Job drawing, mm, ordinate dimensions from the low corner. One solid piece. A direction names the side the tool comes from. Give positions to 0.01 mm unless a question says otherwise; leave off trailing zeros. Loops run counter-clockwise (first coordinate to the right, second up) from the corner with the lowest first, then second, coordinate; pieces in that order, holes last. Notation, with made-up numbers: M 64,7.5 L 110,7.5 A25 ccw 110,33.5 Z; hole C -34.75,88 d10. An arc over 180 degrees is marked long. Answer as CSV lines item,"result".
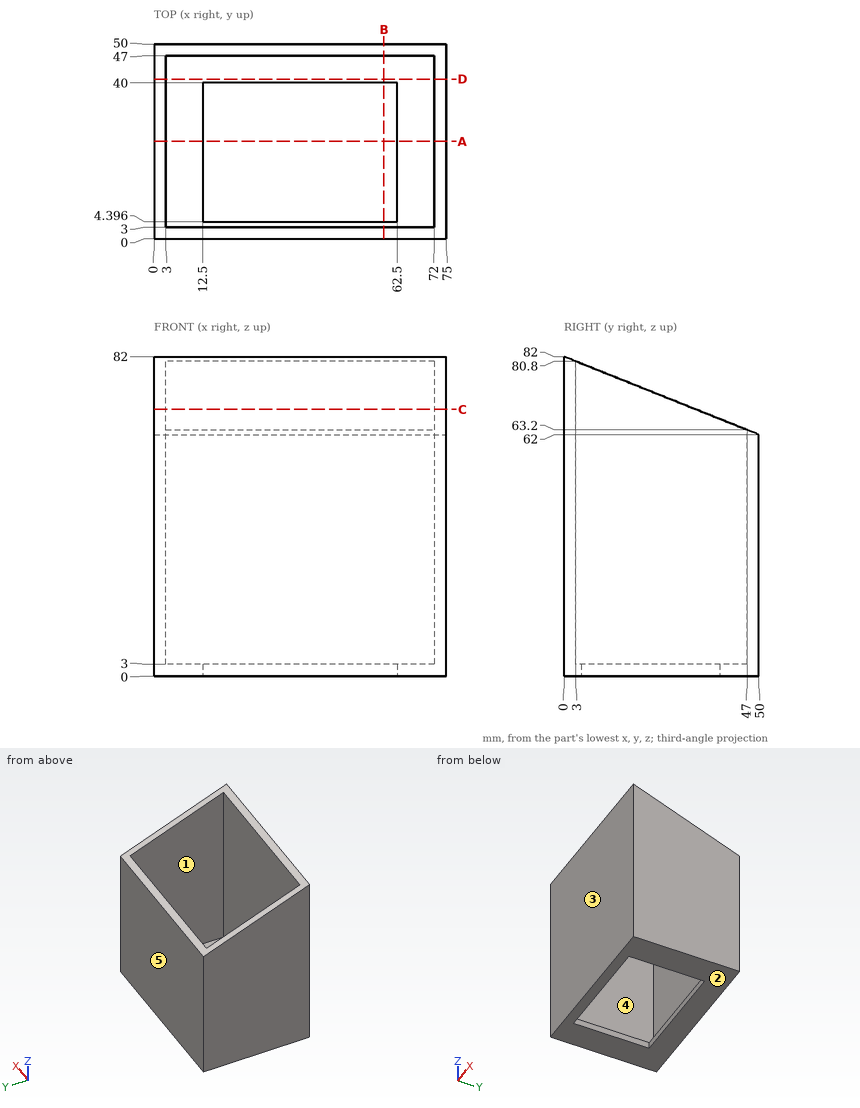
1) Mould opens along Y. For the marked faces 1, 2 and 3 say: +Y half, -Y half, draft (parallel to the pull), parting line (faces both ways), or undercut.
Answer below:
face 1,"undercut"
face 2,"draft"
face 3,"-Y half"
2) Band-saw the part on A-A on y = 25. Give the cut face in (x, z).
Answer below:
outline,"M 0,0 L 12.5,0 L 12.5,3 L 3,3 L 3,72 L 0,72 Z; M 62.5,0 L 75,0 L 75,72 L 72,72 L 72,3 L 62.5,3 Z"
3) Which spindle directions (+Z, -Z, +X, -X, +Y, -Y) get a long thin tool onto all of the face, cutting with end or side? Do the marked faces 4 and 5. Say none if no direction does.
Answer below:
face 4,"+Z"
face 5,"+Z, -Z, +X, -X, +Y"
4) Flat gauge pin, fed straight in: pin 1 (12 mm diameter, centred on x = 19.5, y = 28.5, fed in from -Z). Where does the tip first touch, or does it go through?
Answer below:
pin 1,"passes through"
5) Band-saw the part on B-B on x = 59. Give the cut face in (y, z) (1 decimal).
Answer below:
outline,"M 0,0 L 4.4,0 L 4.4,3 L 3,3 L 3,80.8 L 0,82 Z; M 40,0 L 50,0 L 50,62 L 47,63.2 L 47,3 L 40,3 Z"
6) Drill centre lines: line 1 (X direction, y = 37, z = 10); line 2 (Y direction, x = 4, z = 25); line 3 (Y direction, x = 37, z = 70). Where is each one in solid material? Low to high. Write a range as from..to.
Answer below:
line 1,"x = 0..3, 72..75"
line 2,"y = 0..3, 47..50"
line 3,"y = 0..3"
7) Band-saw the part on C-C on z = 68.5. Give the cut face in (x, y).
Answer below:
outline,"M 0,0 L 75,0 L 75,33.75 L 72,33.75 L 72,3 L 3,3 L 3,33.75 L 0,33.75 Z"
8) Band-saw the part on D-D on y = 41. Give the cut face in (x, z).
Answer below:
outline,"M 0,0 L 75,0 L 75,65.6 L 72,65.6 L 72,3 L 3,3 L 3,65.6 L 0,65.6 Z"
